For this review, use the dimensioned drawing (mm, ordinates from the lowest corner) and the shaded views. A direction names the side the tool comes from. Round coordinates to 2 decimals unless told otherwise and drop trailing zeros. Loops run counter-clockwise (first coordinate to the right, second up) from the corner with the lowest first, then second, coordinate; pieces in that order, holes last.
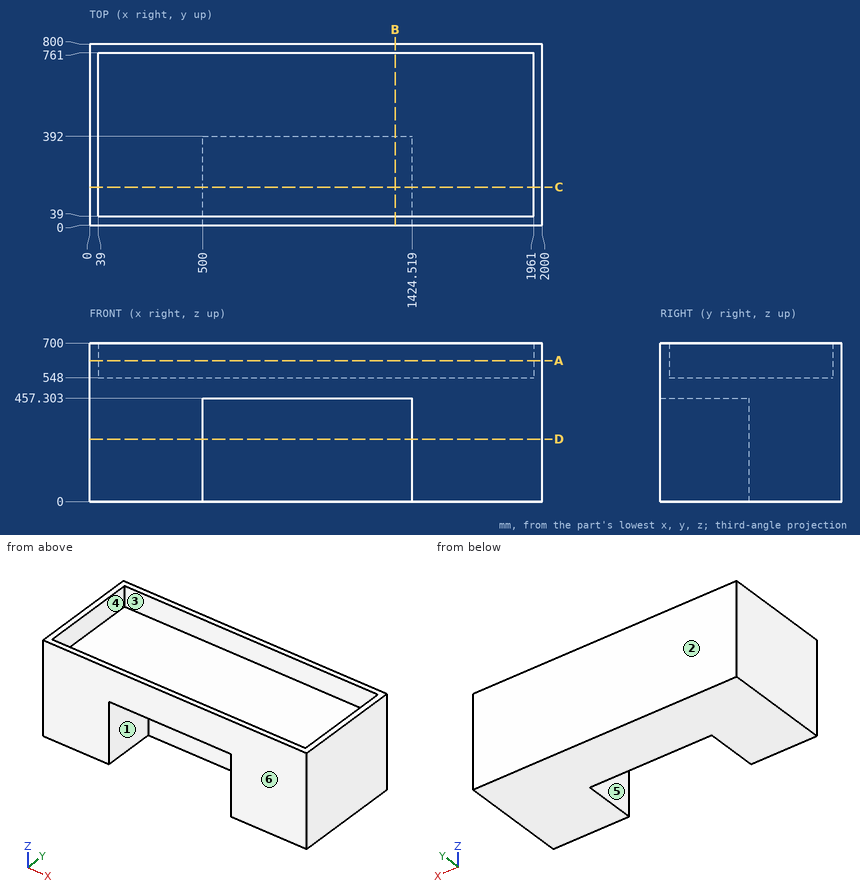
(1) Insertion check: pin 1 Ø1.5 at (x, y) = (1677, 713.5) entering from +Z; pin 2 Ø10 at (x, z) = (1037, 199.5) entering from -Y; pin 3 Ø1 at (x, y) = (603.5, 184) entering from -Z. Each pin has a flat end and moves straight along its axis. Give the tip position at first contact, or say it passes through.
(2) Add section A-A (z = 623). Give the boundary of the cut face in (x, y).
(3) The part is to be moulded in two halves that separate along Y. For the marked faces 4, 5 and 6, say which applies: pulls with the +Y half, pulls with the -Y half, needs draft (parallel to the pull), parting line crosses it, or undercut.
(4) Add section D-D (z = 276.5). Give the boundary of the cut face in (x, y), plus the area to 3 significant figures.
(5) For the marked faces 1, 2 and 3, list the 3-axis set-ups (+Z, -Z, +X, -X, +Y, -Y) from which the entire face can be reached by the end or side of a thin tool; tool diameter is ignored.
(6) Add section B-B (x = 1350). Give the boundary of the cut face in (y, z).
(7) Add section C-C (y = 168). Give the boundary of the cut face in (x, z).
(8) For L1, parallel to X at y = 126.5, z = 570.5; L2, parallel to Y at x = 833.5, z = 665; L3, parallel to X at y = 372, z = 443, list the stretches that pass through material, from the lowest coordinate up.
Outcome:
1. pin 1: stops at z = 548
1. pin 2: stops at y = 392
1. pin 3: stops at z = 457.3
2. outline: (0, 0) - (2000, 0) - (2000, 800) - (0, 800) - close; hole (39, 39) - (1961, 39) - (1961, 761) - (39, 761) - close
3. face 4: undercut
3. face 5: needs draft
3. face 6: pulls with the -Y half
4. outline: (0, 0) - (500, 0) - (500, 392) - (1424.52, 392) - (1424.52, 0) - (2000, 0) - (2000, 800) - (0, 800) - close
4. area: 1,240,000 mm2
5. face 1: -Z, -Y
5. face 2: +Z, -Z, +X, -X, +Y
5. face 3: +Z
6. outline: (0, 457.3) - (392, 457.3) - (392, 0) - (800, 0) - (800, 700) - (761, 700) - (761, 548) - (39, 548) - (39, 700) - (0, 700) - close
7. outline: (0, 0) - (500, 0) - (500, 457.3) - (1424.52, 457.3) - (1424.52, 0) - (2000, 0) - (2000, 700) - (1961, 700) - (1961, 548) - (39, 548) - (39, 700) - (0, 700) - close
8. L1: x = 0 to 39, 1961 to 2000
8. L2: y = 0 to 39, 761 to 800
8. L3: x = 0 to 500, 1424.52 to 2000
